Autodesk Fusion 360 part; units mm, degrees
sketch "Sketch1" plane through (0, 0, 0) normal (0, 1, 0) x (1, 0, 0)
  circle A0 centre (0, 0) radius 35
  circle A1 centre (25, 0) radius 1.5
  line L0 (0, 0) -> (25, 0)
  circle A2 centre (0, 25) radius 1.5
  circle A3 centre (-25, 0) radius 1.5
  circle A4 centre (0, -25) radius 1.5
  circle A5 centre (0, 0) radius 4
  circle A6 centre (-25, 0) radius 4
  circle A7 centre (0, 25) radius 4
  circle A8 centre (25, 0) radius 4
  circle A9 centre (0, -25) radius 4
  dimension "d1" = 70
  dimension "d2" = 3
  dimension "d3" = 25
  dimension "d5" = 360
  dimension "d6" = 8
  dimension "d21" = 8
  dimension "d22" = 8
  dimension "d23" = 8
  dimension "d24" = 8
sketch "Sketch3" plane through (0, 0, 0) normal (0, 0, 1) x (1, 0, 0)
  line L0 (0, 0) -> (0, 70)
  line L1 (0, 0) -> (35, 0)
  line L2 (35, 0) -> (0, 70)
  dimension "d18" = 70
  dimension "d19" = 35
revolve "Revolve1" add sketch "Sketch3" angle 360 about axis through (0, 0, 0) along (0, 1, 0)
extrude "Extrude4" add sketch "Sketch1" along normal blind 7 contours A5
extrude "Extrude6" cut sketch "Sketch1" along normal blind 30 contours A1 | A8 | A2 | A3 | A4 | A6 | A7 | A9
extrude "Extrude7" add sketch "Sketch1" along normal blind 7 contours A8 | A6 | A7 | A9
extrude "Extrude8" cut sketch "Sketch1" along normal blind 70 contours A5
extrude "Extrude9" add sketch "Sketch1" along normal blind 1 contours A5
sketch "Sketch4" plane through (0, 0, 0) normal (0, 0, 1) x (1, 0, 0)
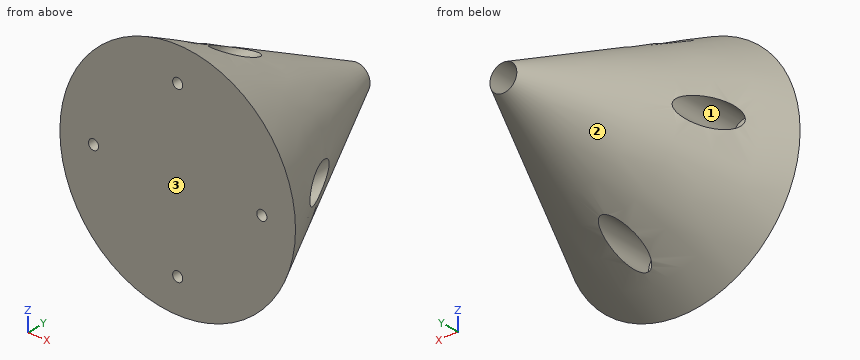
Geometry check sheet. Reference: the model listing, model coordinates, mm. Face numbers are marked on the shaded views. Coordinates: 2 decimals unless noted, no trailing zeros. Order: outer loops, then holes, each group sorted by start corner. A loop starts at its lowest first (then second) coordinate and runs counter-clockwise, first axis right, second up. Notation, with made-up numbers: (-1, 71.5) - (9, 71.5) arc R30 cw to (9, 96.5) - close; hole circle Ø6 at (65, 2). An arc over 180 degrees is marked (long way). Answer in a Markdown table with one row per item. Add a question column.
1) Material ranges on line 1 along X through (y, z) = (4.25, 0) (3 decimals); line 2 along Z through (x, y) = (0, 15.25); line 3 along Z through (x, y) = (25, 3), recorded low to high. Write a range as [from, to].
2) Cross-section at B-B, the plane y = 8.5. Record the cut outline in (x, z), then the cut area to 3 significant figures.
3) Cross-section at D-D, the plane x = -0.5. State how many separate pieces and enclosed holes the cut face has, then the cut area to 3 significant figures.
4) Release check for a two-part mould opening along Z. For the marked faces 1, 2 and 3 record: +Z half, -Z half, draft (parallel to the pull), parting line (faces both ways), or undercut.
5) Cross-section at C-C, the plane y = 17. Record the cut outline in (x, z) (3 decimals).
6) Cross-section at A-A, the plane z = 0. Record the cut outline in (x, y).
7) Gauge pin test, flat ends, axial feed: P1, Ø5, axis at x = 0, z = 0, coming from the +Y side; P2, Ø10, axis at y = 8.5, z = -16, coming from the -X side; P3, Ø9, axis at x = 0, z = -25, coming from the +Y side; P4, Ø9, axis at x = 0, z = 25, coming from the -Y side. Record the tip position at first contact, or that the pin passes through.
Check result:
| question | item | result |
|---|---|---|
| 1 | line 1 | x = [-32.875, -26.5], [-23.5, -4], [4, 23.5], [26.5, 32.875] |
| 1 | line 2 | z = [-21, -4], [4, 21] |
| 1 | line 3 | z = [-22.3, -1.5], [1.5, 22.3] |
| 2 | outline | circle Ø61.5 at (0, 0); hole circle Ø8 at (-25, 0); hole circle Ø8 at (0, -25); hole circle Ø8 at (0, 0); hole circle Ø8 at (0, 25); hole circle Ø8 at (25, 0) |
| 2 | area | 2,720 mm² |
| 3 | separate pieces | 3 |
| 3 | enclosed holes | 0 |
| 3 | area | 1,690 mm² |
| 4 | face 1 | undercut |
| 4 | face 2 | parting line |
| 4 | face 3 | draft |
| 5 | outline | (-26.225, -3.808) arc R26.5 ccw to (-3.808, -26.225) arc R4 cw (long way) to (3.808, -26.225) arc R26.5 ccw to (26.225, -3.808) arc R4 cw (long way) to (26.225, 3.808) arc R26.5 ccw to (3.808, 26.225) arc R4 cw (long way) to (-3.808, 26.225) arc R26.5 ccw to (-26.225, 3.808) arc R4 cw (long way) to start; hole circle Ø8 at (0, 0) |
| 6 | outline | (-35, 0) - (-26.5, 0) - (-26.5, 7) - (-29, 7) - (-29, 12) - close; (-23.5, 0) - (23.5, 0) - (23.5, 7) - (21, 7) - (21, 28) - (4, 62) - (4, 1) - (-4, 1) - (-4, 62) - (-21, 28) - (-21, 7) - (-23.5, 7) - close; (26.5, 0) - (35, 0) - (29, 12) - (29, 7) - (26.5, 7) - close |
| 7 | P1 | stops at y = 1 |
| 7 | P2 | stops at x = -30.06 |
| 7 | P3 | stops at y = 29 |
| 7 | P4 | stops at y = 0 |
